Answer from the drawing. Dimensions are ordinates in mm from the lowest x, y and z of the part. A direction names the side the tool comes from. Coordinates: 2 decimals unless noted, no trailing zeros. Loops run counter-clockwise (first coordinate to the right, second up) from the corner with the lowest first, then second, coordinate; pieces in that order, holes last. Notation, with made-up numbers: M 23,69 L 60,69 A25 ccw 60,103 Z; hole C -31,83 d11. An arc over 180 degrees is marked long. Answer as CSV lines item,"result". Start each with the question number.
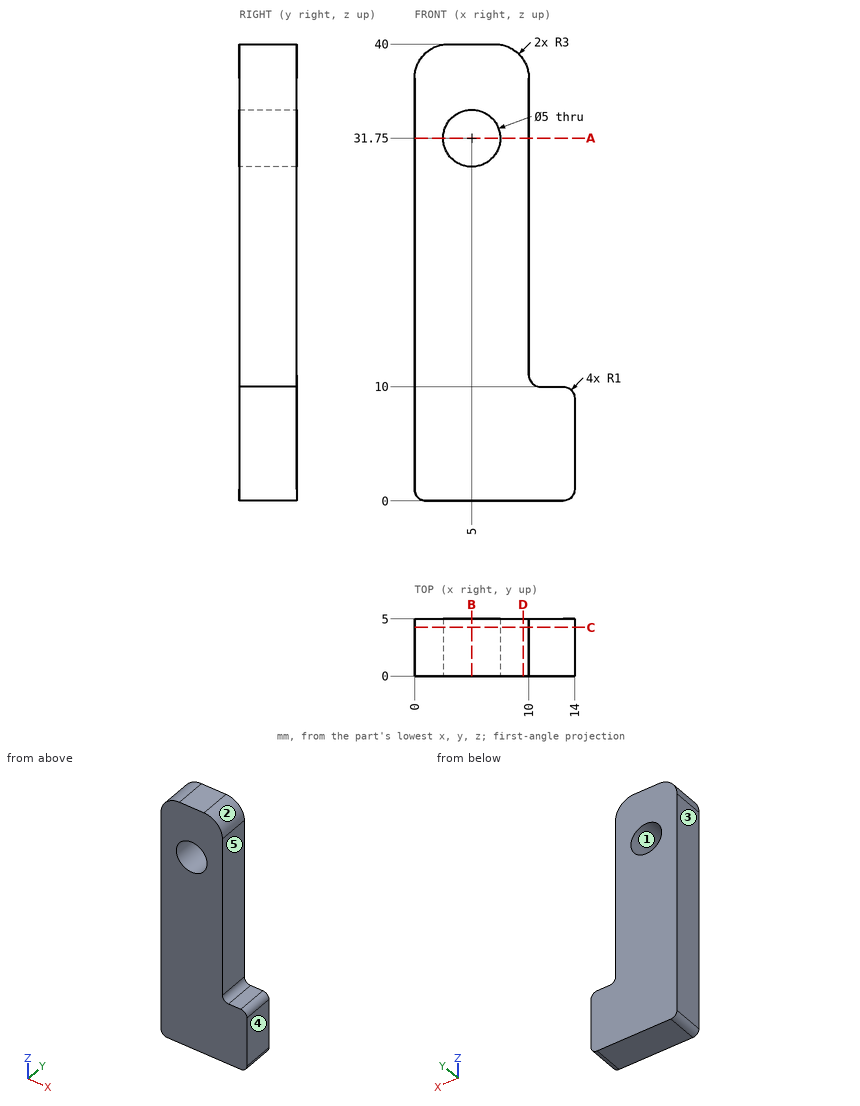
Item 1: Consider line 1 (X direction, y = 3.6, z = 31.75); line 2 (X direction, y = 4.15, z = 21); line 3 (Z direction, x = 4.5, y = 1.25). Determine where each line is inside the solid, lowest interval first.
Item 2: Section C-C on y = 4.25 is taken. Determine the outline of the cut face in (x, z), then the cut area to 3 significant figures.
Item 3: Section A-A on z = 31.75 is taken. Determine the outline of the cut face in (x, y), then the cut area to 3 significant figures.
Item 4: Section B-B on x = 5 is taken. Determine the outline of the cut face in (y, z).
Item 5: For a pull along Z with two mould halves and no side action, classify the marked faces 1, 2 and 3 as pulls with the +Z half, pulls with the -Z half, needs draft (parallel to the pull), parting line crosses it, or undercut.
Item 6: For the marked faces 4 and 5, determine the directions among +Z, -Z, +X, -X, +Y, -Y from which every point of the face is accessible in a straight line to the end or side of a thin tool.
Item 7: Each of these flat-tipped pins is pushed along its axis until it touches: P1, Ø0.6, axis at x = 12, y = 2, coming from the +Z side; P2, Ø2, axis at x = 10, y = 1.5, coming from the +Z side; P3, Ø1.5, axis at x = 12, z = 25.5, coming from the +Y side. Where does it stop, or does it pass through?
Item 8: Section D-D on x = 9.5 is taken. Determine the outline of the cut face in (y, z), then the cut area to 3 significant figures.
Results are:
1,line 1,"0 to 2.5, 7.5 to 10"
1,line 2,"0 to 10"
1,line 3,"0 to 29.3, 34.2 to 40"
2,outline,"M 0,1 A1 ccw 1,0 L 13,0 A1 ccw 14,1 L 14,9 A1 ccw 13,10 L 11,10 A1 cw 10,11 L 10,37 A3 ccw 7,40 L 3,40 A3 ccw 0,37 Z; hole C 5,31.75 d5"
2,area,"416 mm²"
3,outline,"M 0,0 L 2.5,0 L 2.5,5 L 0,5 Z; M 7.5,0 L 10,0 L 10,5 L 7.5,5 Z"
3,area,"25.0 mm²"
4,outline,"M 0,0 L 5,0 L 5,29.25 L 0,29.25 Z; M 0,34.25 L 5,34.25 L 5,40 L 0,40 Z"
5,face 1,"undercut"
5,face 2,"pulls with the +Z half"
5,face 3,"needs draft"
6,face 4,"+Z, -Z, +X, +Y, -Y"
6,face 5,"+Z, +X, +Y, -Y"
7,P1,"z = 10"
7,P2,"z = 39.24"
7,P3,"through"
8,outline,"M 0,0 L 5,0 L 5,38.66 L 0,38.66 Z"
8,area,"193 mm²"
